from build123d import *

# Parameters (mm, degrees)
BOSS_EXTRUDE1_DEPTH      = 32
SKETCH1_3_R              = 16
SKETCH1_3_R_2            = 5
BOSS_EXTRUDE2_DEPTH      = 12
SKETCH1_4_R              = 29
SKETCH1_4_R_2            = 2.65
SKETCH1_4_R_3            = 16
BOSS_EXTRUDE3_DEPTH      = 6
SKETCH1_5_R              = 29
SKETCH1_5_R_2            = 16
SKETCH1_5_R_3            = 5
BOSS_EXTRUDE4_DEPTH      = 56
BOSS_EXTRUDE5_DEPTH      = 12
BOSS_EXTRUDE5_DEPTH_BACK = 5
SKETCH3_R                = 9.808050829
BOSS_EXTRUDE6_DEPTH      = 7
FILLET1_R                = 3


with BuildPart() as part:
    # Sketch1 → Boss-Extrude1 (new body)
    with BuildSketch(Plane(origin=(0, 0, 0), x_dir=(1, 0, 0), z_dir=(0, 1, 0))):
        with BuildLine():
            Line((-3.535533906, 3.535533906), (-3.535533906, -3.535533906))
            ThreePointArc((-3.535533906, -3.535533906), (1.913417162, -4.619397663), (5, 0))
            ThreePointArc((5, 0), (1.913417162, 4.619397663), (-3.535533906, 3.535533906))
        make_face()
    extrude(amount=BOSS_EXTRUDE1_DEPTH)

    # Sketch1_3 → Boss-Extrude2 (add)
    with BuildSketch(Plane(origin=(0, 0, 0), x_dir=(1, 0, 0), z_dir=(0, 1, 0))):
        with Locations(Location((0, 0, 0), (0, 0, 270))):
            Circle(SKETCH1_3_R)
        Circle(SKETCH1_3_R_2, mode=Mode.SUBTRACT)
        with BuildLine():
            Line((-3.535533906, 3.535533906), (-3.535533906, -3.535533906))
            ThreePointArc((-3.535533906, -3.535533906), (1.913417162, -4.619397663), (5, 0))
            ThreePointArc((5, 0), (1.913417162, 4.619397663), (-3.535533906, 3.535533906))
        make_face()
        with BuildLine():
            ThreePointArc((-3.535533906, 3.535533906), (-5, 0), (-3.535533906, -3.535533906))
            Line((-3.535533906, -3.535533906), (-3.535533906, 3.535533906))
        make_face()
    extrude(amount=BOSS_EXTRUDE2_DEPTH)

    # Sketch1_4 → Boss-Extrude3 (add)
    with BuildSketch(Plane(origin=(0, 0, 0), x_dir=(1, 0, 0), z_dir=(0, 1, 0))):
        with BuildLine():
            Line((-28.75, 31.75), (28.75, 31.75))
            ThreePointArc((28.75, 31.75), (30.871320344, 30.871320344), (31.75, 28.75))
            Line((31.75, 28.75), (31.75, -28.75))
            ThreePointArc((31.75, -28.75), (30.871320344, -30.871320344), (28.75, -31.75))
            Line((28.75, -31.75), (-28.75, -31.75))
            ThreePointArc((-28.75, -31.75), (-30.871320344, -30.871320344), (-31.75, -28.75))
            Line((-31.75, -28.75), (-31.75, 28.75))
            ThreePointArc((-31.75, 28.75), (-30.871320344, 30.871320344), (-28.75, 31.75))
        make_face()
        Circle(SKETCH1_4_R, mode=Mode.SUBTRACT)
        with Locations(Location((-26.2, 26.2, 0), (0, 0, 270))):
            Circle(SKETCH1_4_R_2, mode=Mode.SUBTRACT)
        with Locations(Location((26.2, 26.2, 0), (0, 0, 270))):
            Circle(SKETCH1_4_R_2, mode=Mode.SUBTRACT)
        with Locations(Location((26.2, -26.2, 0), (0, 0, 270))):
            Circle(SKETCH1_4_R_2, mode=Mode.SUBTRACT)
        with Locations(Location((-26.2, -26.2, 0), (0, 0, 270))):
            Circle(SKETCH1_4_R_2, mode=Mode.SUBTRACT)
        Circle(SKETCH1_4_R)
        with Locations(Location((0, 0, 0), (0, 0, 270))):
            Circle(SKETCH1_4_R_3, mode=Mode.SUBTRACT)
    extrude(amount=BOSS_EXTRUDE3_DEPTH)

    # Sketch1_5 → Boss-Extrude4 (add)
    with BuildSketch(Plane(origin=(0, 0, 0), x_dir=(1, 0, 0), z_dir=(0, 1, 0))):
        with Locations(Location((0, 0, 0), (0, 0, 270))):
            Circle(SKETCH1_5_R)
        with Locations(Location((0, 0, 0), (0, 0, 270))):
            Circle(SKETCH1_5_R_2, mode=Mode.SUBTRACT)
        with Locations(Location((0, 0, 0), (0, 0, 270))):
            Circle(SKETCH1_5_R_2)
        Circle(SKETCH1_5_R_3, mode=Mode.SUBTRACT)
        with BuildLine():
            ThreePointArc((-3.535533906, 3.535533906), (-5, 0), (-3.535533906, -3.535533906))
            Line((-3.535533906, -3.535533906), (-3.535533906, 3.535533906))
        make_face()
        with BuildLine():
            Line((-3.535533906, 3.535533906), (-3.535533906, -3.535533906))
            ThreePointArc((-3.535533906, -3.535533906), (1.913417162, -4.619397663), (5, 0))
            ThreePointArc((5, 0), (1.913417162, 4.619397663), (-3.535533906, 3.535533906))
        make_face()
    extrude(amount=-BOSS_EXTRUDE4_DEPTH)

    # Sketch2 → Boss-Extrude5 (add, two sides)
    with BuildSketch(Plane.ZY.offset(28.869533834)) as boss_extrude5_sk:
        Polygon((-1.063399037, -56), (4.330127019, -56), (7.026890047, -51.32906942), (6.838640743, -50.536822393), (7.618871446, -50.303727559), (10.315634474, -45.632796979), (7.618871446, -40.961866399), (6.838640743, -40.728771565), (7.026890047, -39.936524538), (4.330127019, -35.265593958), (-1.063399037, -35.265593958), (-1.655380436, -35.82474615), (-2.247361835, -35.265593958), (-7.640887891, -35.265593958), (-10.337650919, -39.936524538), (-10.149401615, -40.728771565), (-10.929632318, -40.961866399), (-13.626395346, -45.632796979), (-10.929632318, -50.303727559), (-10.149401615, -50.536822393), (-10.337650919, -51.32906942), (-7.640887891, -56), (-2.247361835, -56), (-1.655380436, -55.440847807), align=None)
    extrude(amount=BOSS_EXTRUDE5_DEPTH)
    extrude(boss_extrude5_sk.sketch, amount=-BOSS_EXTRUDE5_DEPTH_BACK)

    # Sketch3 → Boss-Extrude6 (add)
    with BuildSketch(Plane.ZY.offset(40.869533834)):
        with Locations(Location((-1.655380436, -45.632796979, 0), (0, 0, 270))):
            Circle(SKETCH3_R)
    extrude(amount=BOSS_EXTRUDE6_DEPTH)

    # Fillet1
    fillet1_edges = [part.edges().sort_by_distance(p)[0] for p in [
        (-47.869533834, -35.82474615, -1.655380436),
    ]]
    fillet(fillet1_edges, radius=FILLET1_R)


solid = part.part
Check sheet for the modelled part. Datum: model origin and axes. Units: mm. A direction names the side the tool comes from. Round coordinates to 2 decimals unless told otherwise and drop trailing zeros. Write each loop counter-clockwise with the first axis right and the second up, starting at its lowest first coordinate (ties: lowest second). Pieces come first, ordered by that corner, then holes. Notation, with made-up numbers: (65.25, 14.25) - (116.25, 14.25) arc R19 ccw to (116.25, 34.25) - close; hole circle Ø5 at (88, 14.25). An arc over 180 degrees is marked (long way). Return JSON: item names as keys, results as strings.
Q1. Cross-section at C-C (x = 0). Record the boundary of the cut face in (y, z).
Returned:
{"outline": "(-56, -29) - (0, -29) - (0, -31.75) - (6, -31.75) - (6, -16) - (12, -16) - (12, -5) - (32, -5) - (32, 5) - (12, 5) - (12, 16) - (6, 16) - (6, 31.75) - (0, 31.75) - (0, 29) - (-56, 29) - close"}
Q2. Draft check along X on faces 5 (the cylindrical face through (-30.89, 2.96, -30.85)), 6 (the cylindrical face through (25.19, 2.96, -23.75)), 7 (the cylindrical face through (24.453, -27.608, 15.59)), 8 (the flat face through (-34.41, -53.7, 5.66)). Enter one of: released by +X, released by -X, zero draft, split by the parting line, or undercut.
Returned:
{"face 5": "released by -X", "face 6": "undercut", "face 7": "split by the parting line", "face 8": "zero draft"}
Q3. Cross-section at D-D (y = 17). Record the boundary of the cut face in (x, z), then the cut area to 3 significant figures.
Returned:
{"outline": "(-3.54, -3.54) arc R5 ccw (long way) to (-3.54, 3.54) - close", "area": "71.4 mm²"}
Q4. Cross-section at A-A (x = 26.2). Record the boundary of the cut face in (y, z).
Returned:
{"outline": "(-56, -12.43) - (0, -12.43) - (0, -23.55) - (6, -23.55) - (6, 23.55) - (0, 23.55) - (0, 12.43) - (-56, 12.43) - close; (0, -31.75) - (6, -31.75) - (6, -28.85) - (0, -28.85) - close; (0, 28.85) - (6, 28.85) - (6, 31.75) - (0, 31.75) - close"}
Q5. Access from +Z, -Z, +X, -X, +Y, -Y to the whole of each face (thin tool, end or side, straight path). Record for faces 1 (the flat face through (-33.89, -37.57, -8.97)), 2 (the cylindrical face through (-42.842, -35.834, -1.224)), 3 (the flat face through (-40.87, -54.5, 3.3)), 4 (the flat face through (4, 12, -4)).
Returned:
{"face 1": "-Z, -X", "face 2": "-X", "face 3": "+Z, -X, -Y", "face 4": "+Y"}
Q6. Depth check by flat-ended pin: P1, Ø1.6, axis at y = -52.5, z = 3, coming from the -X side; P2, Ø10, axis at y = 1.5, z = -17, coming from the -X side; P3, Ø7, axis at x = 26.2, z = 26.2, coming from the +Y side. Enter the tip coordinate at first touch or a pass-through.
Returned:
{"P1": "stops at x = -47.79", "P2": "stops at x = -31.75", "P3": "stops at y = 6"}
Q7. Scan lines: L1, parallel to X at y = 3.1, z = -26.2; L2, parallel to Z at x = -26, y = 1; L3, parallel to Y at x = -29, z = 4. Record each from-to range of solid material in increasing order. Write a range as from..to.
Returned:
{"L1": "x = -31.75..-28.85, -23.55..23.55, 28.85..31.75", "L2": "z = -31.75..-28.84, -23.56..23.56, 28.84..31.75", "L3": "y = -56..-35.27, 0..6"}
Q8. Cross-section at B-B (z = 26.2). Record the boundary of the cut face in (x, y).
Returned:
{"outline": "(-31.75, 0) - (-28.85, 0) - (-28.85, 6) - (-31.75, 6) - close; (-23.55, 0) - (-12.43, 0) - (-12.43, -56) - (12.43, -56) - (12.43, 0) - (23.55, 0) - (23.55, 6) - (-23.55, 6) - close; (28.85, 0) - (31.75, 0) - (31.75, 6) - (28.85, 6) - close"}
